Autodesk Inventor part; units mm, degrees
ref_plane "YZ Plane" through (0, 0, 0) normal (1, 0, 0) x (0, 1, 0)
ref_plane "XZ Plane" through (0, 0, 0) normal (0, 1, 0) x (-1, 0, 0)
ref_plane "XY Plane" through (0, 0, 0) normal (0, 0, 1) x (1, 0, 0)
sketch "Sketch1" plane through (0, 0, 0) normal (0, 0, 1) x (1, 0, 0)
  circle A0 centre (0, 0) radius 5
  circle A1 centre (15.45, 0) radius 2.6
  arc A2 (16.1104, -3.7929) -> (16.3595, 3.741) centre (15.45, 0) ccw
  arc A3 (1.7718, 7.2877) -> (-3.175, -6.7948) centre (0, 0) ccw
  line L0 (1.7718, 7.2877) -> (16.3595, 3.741)
  arc A4 (-3.175, -18) -> (3.175, -18) centre (0, -18) ccw
  line L1 (3.175, -18) -> (3.175, -6.045)
  line L2 (-3.175, -6.7948) -> (-3.175, -18)
  line L3 (-20, -8.85) -> (-20, -3.85)
  line L4 (-20, -8.85) -> (-20, -18.85)
  line L5 (-20, -3.85) -> (-4.0301, 6.3252)
  line L6 (-20, -3.85) -> (-6.4364, -3.85)
  line L7 (-20, -18.85) -> (-0.37, -21.1534)
  line L8 (16.1104, -3.7929) -> (3.175, -6.045)
  line L9 (-3.175, -18) -> (-3.175, -20.8242)
  point P0 (-20, -5.6718)
  dimension "d0" = 15.45
  dimension "d1" = 5.2
  dimension "d2" = 10
  dimension "d3" = 0
  dimension "d4" = 7.7
  dimension "d5" = 15
  dimension "d6" = 6.35
  dimension "d7" = 0
  dimension "d9" = 18
  dimension "d21" = 8.85
  dimension "d22" = 20
  dimension "d23" = 5
  dimension "d24" = 10
extrude "Extrusion3" add sketch "Sketch1" along normal blind 3
fillet "Fillet7" radius 2 1 edges at (3.175, -6.045, 1.5)
extrude "Extrusion6" add sketch "Sketch1" against normal blind 12.3 contours A3 L2 L9 L7 L4 L3 L6
sketch "Sketch5" plane through (-20, -18.85, 3) normal (-1, 0, 0) x (0, 0, 1)
  line L0 (-3, 26.35) -> (0, 26.35)
  line L1 (0, 15) -> (0, 0)
  circle A0 centre (-9.15, 10) radius 3.15
  line L2 (-3, -1.9742) -> (-3, 12.0552)
  point P0 (-3, 18.85)
  point P1 (-3, 13.1782)
  point P2 (-3, 10)
  dimension "d43" = 6.3
  dimension "d44" = 0
  dimension "d45" = 6.15
sketch "Sketch6" plane through (0, 0, 3) normal (0, 0, 1) x (1, 0, 0)
  line L0 (-20, -12) -> (-3.175, -12)
  circle A0 centre (0, 0) radius 5
  circle A1 centre (15.45, 0) radius 2.6
  line L1 (-4.0301, 6.3252) -> (-20, -3.85)
  line L2 (-20, -3.85) -> (-20, -18.85)
  line L3 (-20, -18.85) -> (-0.37, -21.1534)
  arc A2 (-0.37, -21.1534) -> (3.175, -18) centre (0, -18) ccw
  line L4 (3.175, -18) -> (3.175, -7.7269)
  arc A3 (4.832, -5.7565) -> (3.175, -7.7269) centre (5.175, -7.7269) ccw
  line L5 (4.832, -5.7565) -> (16.1104, -3.7929)
  arc A4 (16.1104, -3.7929) -> (16.3595, 3.741) centre (15.45, 0) ccw
  line L6 (16.3595, 3.741) -> (1.7718, 7.2877)
  arc A5 (1.7718, 7.2877) -> (-4.0301, 6.3252) centre (0, 0) ccw
  line L7 (-20, -5.7) -> (-4.8744, -5.7)
  line L8 (-3.175, -20.8242) -> (-3.175, -6.7948)
  line L9 (-3.175, -6.7948) -> (-3.175, -20.8242)
  line L10 (-9.175, -18) -> (-6.175, -18)
  line L11 (-6.175, -18) -> (-6.175, -13)
  line L12 (-6.175, -13) -> (-9.175, -13)
  line L13 (-9.175, -13) -> (-9.175, -18)
  dimension "d55" = 5
  dimension "d56" = 3
  dimension "d57" = 3
  dimension "d58" = 1
extrude "Extrusion8" cut sketch "Sketch6" against normal up to next contours L13 L12 L11 L10
fillet "Fillet8" radius 2 1 edges at (-20, -18.85, -4.65)
fillet "Fillet9" radius 2 1 edges at (-20, -3.85, -6.15)
fillet "Fillet10" radius 1 1 edges at (-6.175, -18, -4.65)
fillet "Fillet11" radius 1 1 edges at (-9.175, -18, -4.65)
fillet "Fillet12" radius 1 1 edges at (-9.175, -13, -4.65)
fillet "Fillet13" radius 1 1 edges at (-6.175, -13, -4.65)
fillet "Fillet14" radius 2 1 edges at (-3.175, -20.8242, -6.15)
fillet "Fillet18" radius 2 1 edges at (-20, -3.85, 1.5)
sketch "Sketch8" plane through (0, 0, -12.3) normal (0, 0, -1) x (-1, 0, 0)
  line L0 (18, -3.85) -> (6.4364, -3.85)
  line L1 (6.175, -17) -> (6.175, -14)
  arc A0 (7.175, -13) -> (6.175, -14) centre (7.175, -14) ccw
  line L2 (7.175, -13) -> (8.175, -13)
  arc A1 (9.175, -14) -> (8.175, -13) centre (8.175, -14) ccw
  line L3 (9.175, -14) -> (9.175, -17)
  arc A2 (8.175, -18) -> (9.175, -17) centre (8.175, -17) ccw
  line L4 (8.175, -18) -> (7.175, -18)
  arc A3 (6.175, -17) -> (7.175, -18) centre (7.175, -17) ccw
  arc A4 (3.175, -18.5758) -> (5.4081, -20.5622) centre (5.175, -18.5758) ccw
  line L5 (5.4081, -20.5622) -> (18.2331, -19.0573)
  arc A5 (18.2331, -19.0573) -> (20, -17.071) centre (18, -17.071) ccw
  line L6 (20, -17.071) -> (20, -5.85)
  arc A6 (20, -5.85) -> (18, -3.85) centre (18, -5.85) ccw
  line L7 (18, -3.85) -> (6.4364, -3.85)
  arc A7 (3.175, -6.7948) -> (6.4364, -3.85) centre (0, 0) ccw
  line L8 (3.175, -6.7948) -> (3.175, -18.5758)
  line L9 (19.9944, -5.7) -> (4.8744, -5.7)
  circle A8 centre (0, 0) radius 7.5
  line L10 (3.175, -6.7948) -> (3.175, -3.85)
  line L11 (3.175, -3.85) -> (6.4364, -3.85)
extrude "Extrusion9" add sketch "Sketch8" against normal up to surface (12.3 mm away) contours A7 L10 L11
extrude "Extrusion10" cut sketch "Sketch5" against normal up to next
fillet "Fillet19" radius 2 1 edges at (-3.175, -3.85, -6.15)
properties part number "bowden_tube_holder"
Verification items for the finished model (mm, model axes). A direction names the side the tool comes from. Coordinates: 2 decimals unless noted, no trailing zeros. Write each loop counter-clockwise with the first axis right and the second up, starting at its lowest first coordinate (ties: lowest second). Pieces come first, ordered by that corner, then holes. Notation, with made-up numbers: (15, 76.25) - (52, 76.25) arc R14 ccw to (52, 97.25) - close; hole circle Ø5 at (73, 21.5). An arc over 180 degrees is marked (long way). Answer as a JSON object with one key per item and string values.
(1) Thickness scan on line 1 along X through (y, z) = (-15.5, -2.5) (3 decimals); line 2 along Y through (x, z) = (-8.5, -6.15); line 3 along Y through (x, z) = (-8.75, -6.15). Record the ranges inside material, lowest first.
Report:
{"line 1": "-20 to -9.175, -6.175 to -3.175", "line 2": "-20.2 to -17.95, -13.05 to -12, -5.7 to -3.85", "line 3": "-20.17 to -17.82, -13.18 to -12, -5.7 to -3.85"}
(2) Cross-section at C-C on y = 2. Record the cut outline in (x, z).
Report:
{"outline": "(-10.82, 0) - (-4.58, 0) - (-4.58, 3) - (-10.82, 3) - close; (4.58, 0) - (13.79, 0) - (13.79, 3) - (4.58, 3) - close; (17.11, 0) - (18.74, 0) - (18.74, 3) - (17.11, 3) - close"}
(3) Tool access check on faces 4 (the cylindrical face through (-11.705, -7.904, -3.145)), 5 (the flat face through (-3.175, -14, -6)), 6 (the cylindrical face through (-6.476, -13.285, -4.757)). Record the directions out of +Z, -Z, +X, -X, +Y, -Y that give a thin tool (end or side, any length) a straight path to the whole face; none if there is none.
Report:
{"face 4": "+X, -X", "face 5": "-Z, +X, +Y, -Y", "face 6": "+Z, -Z"}
(4) Cross-section at B-B on z = -6.15. Record the cut outline in (x, y) (3 decimals).
Report:
{"outline": "(-20, -17.071) arc R2 ccw to (-18.233, -19.057) - (-5.408, -20.562) arc R2 ccw to (-3.175, -18.576) - (-3.175, -12) - (-20, -12) - close; (-19.994, -5.7) - (-3.181, -5.7) arc R2 ccw to (-5.175, -3.85) - (-18, -3.85) arc R2 ccw to start; hole (-9.175, -17) arc R1 ccw to (-8.175, -18) - (-7.175, -18) arc R1 ccw to (-6.175, -17) - (-6.175, -14) arc R1 ccw to (-7.175, -13) - (-8.175, -13) arc R1 ccw to (-9.175, -14) - close"}
(5) Cross-section at D-D on x = -15. Record the cut outline in (y, z).
Report:
{"outline": "(-19.44, -12.3) - (-3.85, -12.3) - (-3.85, 0) - (-0.66, 0) - (-0.66, 3) - (-19.44, 3) - close; hole circle Ø6.3 at (-8.85, -6.15)"}
(6) Mould release check, pull along Y, two halves, no side actions. Record for faces 1 (the flat face through (-8, -18, -5)), 2 (the cylindrical face through (2.138, -20.347, 1.479)), 3 (the flat face through (3.175, -13, 1)): pulls with the +Y half, pulls with the -Y half, needs draft (parallel to the pull), parting line crosses it, or undercut.
Report:
{"face 1": "undercut", "face 2": "pulls with the -Y half", "face 3": "needs draft"}
(7) Cross-section at A-A on y = -16.5. Record the cut outline in (x, z) (3 decimals).
Report:
{"outline": "(-20, -12.3) - (-9.175, -12.3) - (-9.175, 3) - (-20, 3) - close; (-6.175, -12.3) - (-3.175, -12.3) - (-3.175, 0) - (3.175, 0) - (3.175, 3) - (-6.175, 3) - close"}
(8) Gauge pin test, flat ends, axial feed: pin 1 Ø3.5 at (y, z) = (-15, -5.5) entering from +X (3 decimals); pin 2 Ø5 at (x, z) = (-2.5, -9) entering from +Y; pin 3 Ø9 at (x, y) = (0, 0) entering from -Z; pin 4 Ø0.8 at (x, z) = (-8, -4) entering from -Y (3 decimals). Record the tip position at first contact, or that the pin passes through.
Report:
{"pin 1": "x = -3.175", "pin 2": "y = -3.86", "pin 3": "through", "pin 4": "y = -20.305"}
